Verification items for the finished model (mm, model axes). A direction names the side the tool comes from. Coordinates: 2 decimals unless noted, no trailing zeros. Loops run counter-clockwise (first coordinate to the right, second up) from the corner with the lowest first, then second, coordinate; pieces in that order, holes last. Notation, with made-up numbers: M -30.5,67 L 27.5,67 A23 ccw 27.5,76 Z; hole C 52.5,54.25 d1. An arc over 180 degrees is marked long. Write item = value, one per line. Start each with the question number.
```python
from build123d import *

# Parameters (mm, degrees)
F1_DEPTH = 0.79375
F2_R     = 0.635


with BuildPart() as f1:
    # F0 (on Front) → F1 (new body, symmetric)
    with BuildSketch(Plane.XZ):
        with BuildLine():
            Line((-6.35, -9.4615), (6.35, -9.4615))
            Line((6.35, -9.4615), (6.35, 9.4615))
            Line((6.35, 9.4615), (-6.35, 9.4615))
            add(Edge.make_bspline(
                [(-6.35, 9.4615), (-9.4238393137, 9.3856386824), (-12.3985658508, 7.064816161), (-15.0919286534, 2.519920934), (-16.51, 0.79375)],
                knots=[0, 0, 0, 0, 0.4891154758, 1, 1, 1, 1], degree=3))
            Line((-16.51, 0.79375), (-3.81, 0.79375))
            Line((-3.81, 0.79375), (-3.81, -0.79375))
            Line((-3.81, -0.79375), (-16.51, -0.79375))
            add(Edge.make_bspline(
                [(-6.35, -9.4615), (-9.4238393137, -9.3856386824), (-12.3985658508, -7.064816161), (-15.0919286534, -2.519920934), (-16.51, -0.79375)],
                knots=[0, 0, 0, 0, 0.4891154758, 1, 1, 1, 1], degree=3))
        make_face()
    extrude(amount=F1_DEPTH, both=True)

    # F2
    f2_edges = [f1.edges().sort_by_distance(p)[0] for p in [
        (6.35, 0, 9.4615),
        (6.35, 0, -9.4615),
    ]]
    fillet(f2_edges, radius=F2_R)


solid = f1.part
```
Q1. Mould release check, pull along Z, two halves, no side actions. Record for faces 3 (the face through (0, 0, -9.462)), 4 (the face through (0, 0, 9.462)), 5 (the face through (-3.81, 0, 0)): +Z half, -Z half, draft (parallel to the pull), parting line (faces both ways), or undercut.
Q2. Scan lines: L1, parallel to Z at x = -6, y = -0.35; L2, parallel to X at y = -0.5, z = 0.25; L3, parallel to Z at x = -13.75, y = -0.2. Record each from-to range of solid material in increasing order. Write a range as [from, to].
Q3. Set-up check for faces 1 (the face through (-10, 0, 0.794)), 2 (the face through (-3, -0.794, 0)): record each of +Z, -Z, +X, -X, +Y, -Y from which the full face is reachable in a straight line by a thin tool's end or side.
Q4. Sectioned sample at B-B on z = -0.5. Record the cut outline in (x, y).
Q5. Sectioned sample at A-A on x = -5. Record the cut outline in (y, z).
Q6. Gauge pin test, flat ends, axial feed: pin 1 (0.5 mm diameter, centred on x = -12, y = 0.5, fed in from -Z); pin 2 (0.5 mm diameter, centred on x = -12.5, y = -0.5, fed in from +Z). Record the tip position at first contact, or that the pin passes through.
Solutions:
q1.face_3 = -Z half
q1.face_4 = +Z half
q1.face_5 = undercut
q2.L1 = [-9.46, -0.79], [0.79, 9.46]
q2.L2 = [-3.81, 6.35]
q2.L3 = [-4.62, -0.79], [0.79, 4.62]
q3.face_1 = -X, +Y, -Y
q3.face_2 = +Z, -Z, +X, -X, -Y
q4.outline = M -3.81,-0.79 L 6.35,-0.79 L 6.35,0.79 L -3.81,0.79 Z
q5.outline = M -0.79,-9.46 L 0.79,-9.46 L 0.79,-0.79 L -0.79,-0.79 Z; M -0.79,0.79 L 0.79,0.79 L 0.79,9.46 L -0.79,9.46 Z
q6.pin_1 = -7.17
q6.pin_2 = 6.6
